Verification items for the finished model (mm, model axes). A direction names the side the tool comes from. Coordinates: 2 decimals unless noted, no trailing zeros. Loops run counter-clockwise (first coordinate to the right, second up) from the corner with the lowest first, then second, coordinate; pieces in that order, holes last. Notation, with made-up numbers: (76, 18) -> (123, 18) arc R7 cw to (123, 28) -> close; hole circle Ø9 at (73, -12.75). An arc over 180 degrees is marked (long way). Answer as a JSON object with one key per item and string values. Group by question number.
Q1. Cross-section at A-A on z = -5.5. Record the boundary of the cut face in (x, y).
Q2. Cross-section at B-B on y = -7. Record the boundary of the cut face in (x, z).
Q3. Scan lines: L1, parallel to Y at x = 0, z = -19.25; L2, parallel to Z at x = -6, y = 3; L3, parallel to Z at x = 5.25, y = -2.75. Record each from-to range of solid material in increasing order.
Q4. Set-up check for faces 1 (the flat face through (-1.048, -1.704, 10.201)), 2 (the cylindrical face through (-0.07, 1.5, -14.7)), 3 (the flat face through (-2, -2, 6)), 4 (the flat face through (3.45, -2.024, 9.549)): record each of +Z, -Z, +X, -X, +Y, -Y from which the full face is reachable in a straight line by a thin tool's end or side.
Q5. Release check for a two-part mould opening along Z. For faces 5 (the flat face through (0.95, 1.76, 10.2)), 6 (the cylindrical face through (0, 0, 17)), 7 (the cylindrical face through (-1.282, 0.773, 12.901)) record: released by +Z, released by -Z, zero draft, split by the parting line, or undercut.
Q6. Gauge pin test, flat ends, axial feed: pin 1 Ø4 at (y, z) = (3, 0) entering from +X; pin 2 Ø2 at (y, z) = (2, 10.5) entering from -X; pin 3 Ø6 at (x, y) = (-4.5, 6.5) entering from +Z. Record the tip position at first contact, or that the pin passes through.
Autodesk Inventor part; units mm, degrees
ref_plane "YZ Plane" through (0, 0, 0) normal (1, 0, 0) x (0, 1, 0)
ref_plane "XZ Plane" through (0, 0, 0) normal (0, 1, 0) x (-1, 0, 0)
ref_plane "XY Plane" through (0, 0, 0) normal (0, 0, 1) x (1, 0, 0)
sketch "スケッチ1" plane through (0, 0, 0) normal (0, 0, 1) x (1, 0, 0)
  line L0 (0, 7.5056) -> (6.5, 3.7528)
  line L1 (6.5, 3.7528) -> (6.5, -3.7528)
  line L2 (6.5, -3.7528) -> (0, -7.5056)
  line L3 (0, -7.5056) -> (-6.5, -3.7528)
  line L4 (-6.5, -3.7528) -> (-6.5, 3.7528)
  line L5 (-6.5, 3.7528) -> (0, 7.5056)
  circle A0 centre (0, 0) radius 6.5
  dimension "d0" = 13
  dimension "d1" = 13
extrude "押し出し1" add sketch "スケッチ1" along normal blind 6
extrude "押し出し2" add sketch "スケッチ1" against normal blind 29 contours A0
ref_plane "作業平面1" through (-3.25, 1.8764, 6) normal (0.5, 0.8660254, 0) x (0.8660254, -0.5, 0)
sketch "スケッチ2" plane through (-3.25, 1.8764, 6) normal (0.5, 0.8660254, 0) x (0.8660254, -0.5, 0)
  line L0 (0, 6) -> (3.7528, 6)
  line L1 (0, 6) -> (0, 0)
  line L2 (7.5056, 0) -> (0, 0)
  line L3 (7.5056, 6) -> (7.5056, 0)
  line L4 (3.7528, 6) -> (3.7528, -7)
  line L5 (3.7528, -7) -> (3.7528, 0) construction
  line L6 (7.7528, -7) -> (7.7528, 0)
  line L7 (-0.2472, 0) -> (-0.2472, -7)
  arc A0 (-0.2472, -7) -> (7.7528, -7) centre (3.7528, -7) ccw
  arc A1 (7.7528, 0) -> (-0.2472, 0) centre (3.7528, 0) ccw
  line L8 (3.7528, 6) -> (7.5056, 6)
  point P0 (3.7528, -3.5)
  dimension "d7" = 7
  dimension "d8" = 8
extrude "押し出し3" add sketch "スケッチ2" along normal mid plane 4 contours A1 L4 L2 L1 | L1 L2 L3 A1 L6 A0 L7 | A1 L3 L2 L4
hole "穴1" at (0, 0, 13) direction (0.5, 0.8660254, 0) diameter 3 end through all
hole "穴2" at (0, 0, 13) direction (-0.5, -0.8660254, 0) diameter 3 end through all
hole "穴3" at (0, 0, 0) direction (0, 0, -1) diameter 3 end through all
sketch "スケッチ3" plane through (0, 0, 6) normal (0, 0, 1) x (1, 0, 0)
  circle A0 centre (0, 0) radius 1.5
  circle A1 centre (0, 0) radius 8
  dimension "d32" = 16
extrude "押し出し4" add sketch "スケッチ3" against normal blind 6
properties part number "ダンパー上パーツ"
Computed values:
{
 "1": {"outline": "circle Ø13 at (0, 0); hole circle Ø3 at (0, 0)"},
 "2": {"outline": "(-3.87, 0) -> (3.87, 0) -> (3.87, 6) -> (-3.87, 6) -> close"},
 "3": {"L1": "y = -6.5 to -1.5, 1.5 to 6.5", "L2": "z = 0 to 6", "L3": "z = -29 to 6"},
 "4": {"face 1": "+Z, -X, -Y", "face 2": "-Z", "face 3": "+Z", "face 4": "+Z, +X, -Y"},
 "5": {"face 5": "zero draft", "face 6": "released by +Z", "face 7": "undercut"},
 "6": {"pin 1": "stops at x = 7.94", "pin 2": "stops at x = -4.04", "pin 3": "stops at z = 6"}
}
